from build123d import *

# Parameters (mm, degrees)
SKETCH1_R               = 25
SKETCH1_W               = 27.5
SKETCH1_H               = 27.5
BOSS_EXTRUDE1_DEPTH     = 55
BOSS_EXTRUDE2_START     = 5
SKETCH2_R               = 25
SKETCH2_W               = 27.5
SKETCH2_H               = 27.5
BOSS_EXTRUDE2_DEPTH     = 5
SKETCH3_W               = 25
SKETCH3_H               = 50
BOSS_EXTRUDE3_DEPTH     = 80
FILLET1_R               = 2.5
FILLET2_R               = 2.5
SKETCH21_W              = 54.3
SKETCH21_H              = 20.3
CUT_EXTRUDE1_DEPTH      = 11.3
SKETCH22_W              = 40.3
SKETCH22_H              = 20.3
CUT_EXTRUDE2_DEPTH      = 93.059763198
CUT_EXTRUDE3_DEPTH      = 88.464278423
SKETCH23_R              = 2.15
CUT_EXTRUDE4_DEPTH      = 93.059763198
CUT_EXTRUDE7_DEPTH      = 27.5
CUT_EXTRUDE8_DEPTH      = 93.059763198
CUT_EXTRUDE8_DEPTH_BACK = 93.059763198
SKETCH25_W              = 77.291444149
SKETCH25_H              = 50
CUT_EXTRUDE9_DEPTH      = 93.059763198
CUT_EXTRUDE9_DEPTH_BACK = 93.059763198
SKETCH26_W              = 62.708555851
SKETCH26_H              = 12.5


with BuildPart() as part:
    # Sketch1 → Boss-Extrude1 (new body)
    with BuildSketch(Plane.XY):
        Circle(SKETCH1_R)
        Rectangle(SKETCH1_W, SKETCH1_H, mode=Mode.SUBTRACT)
    extrude(amount=BOSS_EXTRUDE1_DEPTH)

    # Sketch2 → Boss-Extrude2 (add)
    # profile 1 of 2: a face of its own
    with BuildSketch(Plane(origin=(0, 0, 0), x_dir=(-1, 0, 0), z_dir=(0, 0, -1)).offset(BOSS_EXTRUDE2_START)):
        Circle(SKETCH2_R)
        Rectangle(SKETCH2_W, SKETCH2_H, mode=Mode.SUBTRACT)
    # profile 2 of 2: a face of its own
    with BuildSketch(Plane(origin=(0, 0, 0), x_dir=(-1, 0, 0), z_dir=(0, 0, -1)).offset(BOSS_EXTRUDE2_START)):
        Rectangle(SKETCH2_W, SKETCH2_H)
    extrude(amount=-BOSS_EXTRUDE2_DEPTH)

    # Sketch3 → Boss-Extrude3 (add)
    with BuildSketch(Plane(origin=(0, 0, -5), x_dir=(-1, 0, 0), z_dir=(0, 0, -1))):
        with Locations((12.5, 0)):
            Rectangle(SKETCH3_W, SKETCH3_H)
    extrude(amount=BOSS_EXTRUDE3_DEPTH)

    # Fillet1
    fillet1_edges = [part.edges().sort_by_distance(p)[0] for p in [
        (-13.75, 13.75, 27.5),
        (-13.75, -13.75, 27.5),
        (13.75, -13.75, 27.5),
        (13.75, 13.75, 27.5),
    ]]
    fillet(fillet1_edges, radius=FILLET1_R)

    # Fillet2
    fillet2_edges = [part.edges().sort_by_distance(p)[0] for p in [
        (0, 13.75, 55),
        (-13.75, 0, 55),
        (0, -13.75, 55),
        (13.75, 0, 55),
        (-13.017766953, 13.017766953, 55),
        (-13.017766953, -13.017766953, 55),
        (13.017766953, -13.017766953, 55),
        (13.017766953, 13.017766953, 55),
    ]]
    fillet(fillet2_edges, radius=FILLET2_R)

    # Sketch21 → Cut-Extrude1 (cut)
    with BuildSketch(Plane(origin=(0, 0, 0), x_dir=(0, 0, -1), z_dir=(1, 0, 0))):
        with Locations((51.85, 0)):
            Rectangle(SKETCH21_W, SKETCH21_H)
    extrude(amount=-CUT_EXTRUDE1_DEPTH, mode=Mode.SUBTRACT)

    # Sketch22 → Cut-Extrude2 (cut, through all)
    with BuildSketch(Plane(origin=(0, 0, 0), x_dir=(0, 0, -1), z_dir=(1, 0, 0))):
        with Locations((51.7, 0)):
            Rectangle(SKETCH22_W, SKETCH22_H)
    extrude(amount=-CUT_EXTRUDE2_DEPTH, mode=Mode.SUBTRACT)

    # Sketch18 → Cut-Extrude3 (cut, through all)
    with BuildSketch(Plane.XY.offset(-5)):
        with BuildLine():
            Line((-25, -25), (0, -25))
            ThreePointArc((0, -25), (-17.67766953, -17.67766953), (-25, 0))
            Line((-25, 0), (-25, -25))
        make_face()
        with BuildLine():
            Line((-25, 25), (-25, 0))
            ThreePointArc((-25, 0), (-17.67766953, 17.67766953), (0, 25))
            Line((0, 25), (-25, 25))
        make_face()
    extrude(amount=-CUT_EXTRUDE3_DEPTH, mode=Mode.SUBTRACT)

    # Sketch23 → Cut-Extrude4 (cut, through all)
    with BuildSketch(Plane(origin=(0, 0, 0), x_dir=(0, 0, -1), z_dir=(1, 0, 0))):
        with Locations(Location((27.85, -5.25, 0), (0, 0, 90))):
            Circle(SKETCH23_R)
        with Locations(Location((75.85, 5.25, 0), (0, 0, 90))):
            Circle(SKETCH23_R)
        with Locations(Location((75.85, -5.25, 0), (0, 0, 90))):
            Circle(SKETCH23_R)
        with Locations(Location((27.85, 5.25, 0), (0, 0, 90))):
            Circle(SKETCH23_R)
    extrude(amount=-CUT_EXTRUDE4_DEPTH, mode=Mode.SUBTRACT)

    # Sketch24 → Cut-Extrude7 (cut, symmetric)
    with BuildSketch(Plane(origin=(0, 0, -51.7), x_dir=(-1, 0, 0), z_dir=(0, 0, -1))):
        with BuildLine():
            Line((13.3, 10.15), (13.3, -10.15))
            Line((13.3, -10.15), (22.846826913, -10.15))
            ThreePointArc((22.846826913, -10.15), (25, 0), (22.846826913, 10.15))
            Line((22.846826913, 10.15), (13.3, 10.15))
        make_face()
    extrude(amount=CUT_EXTRUDE7_DEPTH, both=True, mode=Mode.SUBTRACT)

    # Sketch25 → Cut-Extrude8 (cut, two sides: drawn at the far end of the back side and taken through both)
    with BuildSketch(Plane(origin=(0, 0, 0), x_dir=(0, 0, -1), z_dir=(1, 0, 0)).offset(-CUT_EXTRUDE8_DEPTH_BACK)):
        with Locations((-16.354277925, 0)):
            Rectangle(SKETCH25_W, SKETCH25_H)
    extrude(amount=CUT_EXTRUDE8_DEPTH + CUT_EXTRUDE8_DEPTH_BACK, mode=Mode.SUBTRACT)

    # Sketch26 → Cut-Extrude9 (cut, two sides: drawn at the far end of the back side and taken through both)
    with BuildSketch(Plane(origin=(0, 0, 0), x_dir=(0, 0, -1), z_dir=(1, 0, 0)).offset(-CUT_EXTRUDE9_DEPTH_BACK)):
        with Locations((53.645722075, 18.75)):
            Rectangle(SKETCH26_W, SKETCH26_H)
        with Locations((53.645722075, -18.75)):
            Rectangle(SKETCH26_W, SKETCH26_H)
    extrude(amount=CUT_EXTRUDE9_DEPTH + CUT_EXTRUDE9_DEPTH_BACK, mode=Mode.SUBTRACT)


solid = part.part
CAD build for the part. Positions are in the model's coordinates, mm. A direction names the side the tool comes from. Coordinates: 2 decimals unless noted, no trailing zeros. Order: outer loops, then holes, each group sorted by start corner. A loop starts at its lowest first (then second) coordinate and runs counter-clockwise, first axis right, second up.
Item 1: Band-saw the part on C-C on z = -45. List the corners of the cut face in (x, y).
Check sheet entries:
outline: (-22.85, -10.15) arc R25 ccw to (-21.65, -12.5) - (0, -12.5) - (0, -10.15) - close; (-22.85, 10.15) - (0, 10.15) - (0, 12.5) - (-21.65, 12.5) arc R25 ccw to start
Item 2: 3-axis set-ups, long thin cutter, end or side, ignore diameter. For faces 1 (the face through (-11.3, 0, -75)), 2 (the face through (-12, 0, -71.85)), 3 (the face through (-13.3, 0, -76)): which of +Z, -Z, +X, -X, +Y, -Y reach the whole face in a straight line?
Check sheet entries:
face 1: +X
face 2: +X, -X
face 3: -X
Item 3: Pin check, flat tips, straight feed: pin 1 Ø6 at (y, z) = (-1.5, -29.5) entering from -X; pin 2 Ø1 at (y, z) = (10, -53.5) entering from -X; pin 3 Ø5.5 at (y, z) = (-5.25, -75.85) entering from +X. Stop position of each tip, or through.
Check sheet entries:
pin 1: stops at x = -13.3
pin 2: stops at x = -22.85
pin 3: stops at x = -11.3
Item 4: Band-saw the part on B-B on x = -1.75. List the corners of the cut face in (y, z).
Check sheet entries:
outline: (-12.5, -85) - (12.5, -85) - (12.5, -22.29) - (-12.5, -22.29) - close; hole (-10.15, -79) - (10.15, -79) - (10.15, -24.7) - (-10.15, -24.7) - close
Item 5: Drill centre lines: L1, parallel to Z at x = -11.9, y = -5.25; L2, parallel to Z at x = -2.25, y = -8.75; L3, parallel to Z at x = -14.5, y = -7.25. Where is each one in solid material? Low to high.
Check sheet entries:
L1: z = -85 to -78, -73.7 to -71.85, -31.55 to -30, -25.7 to -22.29
L2: z = -85 to -79, -24.7 to -22.29
L3: z = -85 to -79.2, -24.2 to -22.29
Item 6: Band-saw the part on D-D on y = 6. List the corners of the cut face in (x, z).
Check sheet entries:
outline: (-24.27, -85) - (0, -85) - (0, -79) - (-11.3, -79) - (-11.3, -77.86) - (-13.3, -77.86) - (-13.3, -79.2) - (-24.27, -79.2) - close; (-24.27, -24.2) - (-13.3, -24.2) - (-13.3, -25.84) - (-11.3, -25.84) - (-11.3, -24.7) - (0, -24.7) - (0, -22.29) - (-24.27, -22.29) - close; (-13.3, -73.84) - (-11.3, -73.84) - (-11.3, -71.85) - (-13.3, -71.85) - close; (-13.3, -31.55) - (-11.3, -31.55) - (-11.3, -29.86) - (-13.3, -29.86) - close
Item 7: Two-plate mould, pull along Z, no slides. Class faces 4 (the face through (0, -11, -60)), 5 (the face through (-13, 0, -22.291)), 6 (the face through (-19, 0, -79.2)): +Z half, -Z half, draft (parallel to the pull), parting line (faces both ways), or undercut.
Check sheet entries:
face 4: draft
face 5: +Z half
face 6: undercut
Item 8: Band-saw the part on A-A on z = -27.85. List the corners of the cut face in (x, y), plus the area to 3 significant figures.
Check sheet entries:
outline: (-22.85, -10.15) arc R25 ccw to (-21.65, -12.5) - (0, -12.5) - (0, -10.15) - (-11.3, -10.15) - (-11.3, -7.4) - (-13.3, -7.4) - (-13.3, -10.15) - close; (-22.85, 10.15) - (-13.3, 10.15) - (-13.3, 7.4) - (-11.3, 7.4) - (-11.3, 10.15) - (0, 10.15) - (0, 12.5) - (-21.65, 12.5) arc R25 ccw to start; (-13.3, -3.1) - (-11.3, -3.1) - (-11.3, 3.1) - (-13.3, 3.1) - close
area: 128 mm2
